```python
from build123d import *

# Parameters (mm, degrees)
BOSS_EXTRUDE1_DEPTH = 0.8
CUT_EXTRUDE1_START  = -2.6
CUT_EXTRUDE1_DEPTH  = 24.5
SKETCH4_W           = 10.1
SKETCH4_H           = 0.8
BOSS_EXTRUDE2_DEPTH = 2.8


with BuildPart() as part:
    # Sketch1 → Boss-Extrude1 (new body)
    with BuildSketch(Plane(origin=(0, 0, 0), x_dir=(1, 0, 0), z_dir=(0, 1, 0))):
        Polygon((13.478240741, 10.45), (-13.478240741, 10.45), (-13.478240741, -10.45), (13.478240741, -10.45), (13.478240741, -0.35), (-8.221759259, -0.35), (-8.221759259, 0.35), (13.478240741, 0.35), align=None)
    extrude(amount=BOSS_EXTRUDE1_DEPTH)

    # Sketch2 → Cut-Extrude1 (cut)
    with BuildSketch(Plane(origin=(13.478240741, 0, 0), x_dir=(0, 0, -1), z_dir=(1, 0, 0)).offset(CUT_EXTRUDE1_START)):
        Polygon((-7.025, 0.5), (-3.775, 0.5), (-4.525, 0.8), (-6.275, 0.8), align=None)
        Polygon((-7.025, 0.3), (-6.275, 0), (-4.525, 0), (-3.775, 0.3), align=None)
        Polygon((7.025, 0.3), (3.775, 0.3), (4.525, 0), (6.275, 0), align=None)
        Polygon((7.025, 0.5), (6.275, 0.8), (4.525, 0.8), (3.775, 0.5), align=None)
    extrude(amount=-CUT_EXTRUDE1_DEPTH, mode=Mode.SUBTRACT)

    # Sketch4 → Boss-Extrude2 (add)
    with BuildSketch(Plane(origin=(13.478240741, 0, 0), x_dir=(0, 0, -1), z_dir=(1, 0, 0))):
        with Locations((-5.4, 0.4)):
            Rectangle(SKETCH4_W, SKETCH4_H)
        with Locations((5.4, 0.4)):
            Rectangle(SKETCH4_W, SKETCH4_H)
    extrude(amount=BOSS_EXTRUDE2_DEPTH)


solid = part.part
```
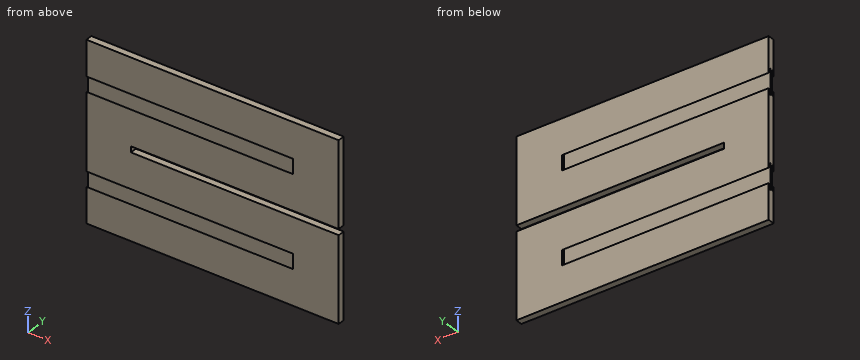
CAD build for the part. Positions are in the model's coordinates, mm. Coordinates: 2 decimals unless noted, no trailing zeros. Order: outer loops, then holes, each group sorted by start corner. A loop starts at its lowest first (then second) coordinate and runs counter-clockwise, first axis right, second up. Notation, with made-up numbers: (37.25, -5.75) - (71.25, -5.75) arc R28 cw to (71.25, 24.25) - close; hole circle Ø7 at (-31.5, -14.75). An arc over 180 degrees is marked (long way). Answer in a Markdown table with one row per item.
1. Drill centre lines: L1, parallel to Z at x = 9.5, y = 0.45; L2, parallel to X at y = 0.65, z = 5.5; L3, parallel to Y at x = 3.75, z = 6. Where is each one in solid material? Low to high. Write a range as from..to.
Answer:
| item | result |
|---|---|
| L1 | -10.45..-0.35, 0.35..10.45 |
| L2 | 10.88..16.28 |
| L3 | 0.3..0.5 |
2. Slice it at B-B, the plane x = -11. List the corners of the cut face in (y, z) (3 decimals), then the cut area to 3 significant figures.
Answer:
| item | result |
|---|---|
| outline | (0, -10.45) - (0.8, -10.45) - (0.8, -6.275) - (0.5, -7.025) - (0.5, -3.775) - (0.8, -4.525) - (0.8, 4.525) - (0.5, 3.775) - (0.5, 7.025) - (0.8, 6.275) - (0.8, 10.45) - (0, 10.45) - (0, 6.275) - (0.3, 7.025) - (0.3, 3.775) - (0, 4.525) - (0, -4.525) - (0.3, -3.775) - (0.3, -7.025) - (0, -6.275) - close |
| area | 13.7 mm² |
3. Slice it at A-A, the plane x = 2. List the corners of the cut face in (y, z) (3 decimals).
Answer:
| item | result |
|---|---|
| outline | (0, -10.45) - (0.8, -10.45) - (0.8, -6.275) - (0.5, -7.025) - (0.5, -3.775) - (0.8, -4.525) - (0.8, -0.35) - (0, -0.35) - (0, -4.525) - (0.3, -3.775) - (0.3, -7.025) - (0, -6.275) - close; (0, 0.35) - (0.8, 0.35) - (0.8, 4.525) - (0.5, 3.775) - (0.5, 7.025) - (0.8, 6.275) - (0.8, 10.45) - (0, 10.45) - (0, 6.275) - (0.3, 7.025) - (0.3, 3.775) - (0, 4.525) - close |
4. Flat gauge pin, fed straight in: P1, Ø1, axis at x = -6.5, z = 5.5, coming from the -Y side. Where does the tip first touch, or does it go through?
Answer:
| item | result |
|---|---|
| P1 | y = 0.3 |
5. Slice it at C-C, the plane x = 12. List the corners of the cut face in (y, z), then the cut area to 3 significant figures.
Answer:
| item | result |
|---|---|
| outline | (0, -10.45) - (0.8, -10.45) - (0.8, -0.35) - (0, -0.35) - close; (0, 0.35) - (0.8, 0.35) - (0.8, 10.45) - (0, 10.45) - close |
| area | 16.2 mm² |
